from build123d import *

# Parameters (mm, degrees)
F1_DEPTH = 2
F2_DEPTH = 3
F3_R     = 8.2
F4_DEPTH = 7.5
F5_R     = 8.2
F5_R_2   = 7
F6_DEPTH = 20
F7_R     = 9
F7_R_2   = 7
F8_DEPTH = 6.5


with BuildPart() as f1:
    # F0 (on Top) → F1 (new body)
    with BuildSketch(Plane.XY):
        with BuildLine():
            Line((0, 9), (0, 10))
            ThreePointArc((0, 10), (-10, 0), (0, -10))
            Line((0, -10), (0, -9))
            ThreePointArc((0, -9), (-9, 0), (0, 9))
        make_face()
    extrude(amount=F1_DEPTH)

    # F0 (on Top) → F2 (join)
    with BuildSketch(Plane.XY):
        with BuildLine():
            ThreePointArc((0, -10), (7.0710678119, -7.0710678119), (10, 0))
            ThreePointArc((10, 0), (7.0710678119, 7.0710678119), (0, 10))
            Line((0, 10), (0, 9))
            ThreePointArc((0, 9), (6.3639610307, 6.3639610307), (9, 0))
            ThreePointArc((9, 0), (6.3639610307, -6.3639610307), (0, -9))
            Line((0, -9), (0, -10))
        make_face()
    extrude(amount=F2_DEPTH)

    # F3 (on face) → F4 (join)
    with BuildSketch(Plane.XY.offset(2)):
        with BuildLine():
            Line((0, 9), (0, 10))
            ThreePointArc((0, 10), (-10, 0), (0, -10))
            Line((0, -10), (0, -9))
            ThreePointArc((0, -9), (-9, 0), (0, 9))
        make_face()
        with BuildLine():
            ThreePointArc((0, -10), (7.0710678119, -7.0710678119), (10, 0))
            ThreePointArc((10, 0), (7.0710678119, 7.0710678119), (0, 10))
            Line((0, 10), (0, 9))
            ThreePointArc((0, 9), (-9, 0), (0, -9))
            Line((0, -9), (0, -10))
        make_face()
        Circle(F3_R, mode=Mode.SUBTRACT)
    extrude(amount=F4_DEPTH)

    # F5 (on face) → F6 (join)
    with BuildSketch(Plane.XY.offset(9.5)):
        Circle(F5_R)
        Circle(F5_R_2, mode=Mode.SUBTRACT)
    extrude(amount=-F6_DEPTH)

    # F7 (on face) → F8 (cut)
    with BuildSketch(Plane.XY.offset(9.5)):
        Circle(F7_R)
        Circle(F7_R_2, mode=Mode.SUBTRACT)
    extrude(amount=-F8_DEPTH, mode=Mode.SUBTRACT)


solid = f1.part
Design review of the part built by this model. Coordinates are the model's own, in mm. A direction names the side the tool comes from. Coordinates: 2 decimals unless noted, no trailing zeros. Write each loop counter-clockwise with the first axis right and the second up, starting at its lowest first coordinate (ties: lowest second). Pieces come first, ordered by that corner, then holes. Notation, with made-up numbers: (52, -19.5) - (90, -19.5) arc R19 cw to (90, 8.5) - close; hole circle Ø3 at (79.25, -34.5). An arc over 180 degrees is marked (long way). Use one line per item in the form item = value.
Q1. Consider section D-D (z = 7). Write out the cut boundary in (x, y), plus the area to 3 significant figures.
Taken from the geometry:
outline = circle Ø20 at (0, 0); hole circle Ø18 at (0, 0)
area = 59.7 mm^2
Q2. Consider section A-A (z = 1.5). Write out the cut boundary in (x, y).
Taken from the geometry:
outline = circle Ø20 at (0, 0); circle Ø16.4 at (0, 0); hole circle Ø18 at (0, 0); hole circle Ø14 at (0, 0)
Q3. The part is to be moulded in two halves that separate along X. For faces 1 (the flat face through (0, -7.3, 3)), 2 (the cylindrical face through (6.466, -2.681, -3.656)), 3 (the flat face through (-9, 2, 9.5)), 4 (the cylindrical face through (9.54, 3, 4.68)), say which applies: +X half, -X half, draft (parallel to the pull), parting line (faces both ways), or undercut.
Taken from the geometry:
face_1 = undercut
face_2 = undercut
face_3 = draft
face_4 = parting line
Q4. For probe 1 along Y at (x, z) = (0, -2.25); probe 2 along X at (y, z) = (-5.5, 1.5); probe 3 along X at (y, z) = (0.5, 1.75), list the stretches that pass through material, from the lowest coordinate up.
Taken from the geometry:
probe_1 = -8.2 to -7, 7 to 8.2
probe_2 = -8.35 to -7.12, -6.08 to -4.33, 4.33 to 6.08, 7.12 to 8.35
probe_3 = -9.99 to -8.99, -8.18 to -6.98, 6.98 to 8.18, 8.99 to 9.99
Q5. Consider section C-C (y = -1.25). Write out the cut boundary in (x, z), plus the area to 3 significant figures.
Taken from the geometry:
outline = (-9.92, 0) - (-8.91, 0) - (-8.91, 2) - (-8.1, 2) - (-8.1, -10.5) - (-6.89, -10.5) - (-6.89, 3) - (-8.91, 3) - (-8.91, 9.5) - (-9.92, 9.5) - close; (6.89, -10.5) - (8.1, -10.5) - (8.1, 2) - (8.91, 2) - (8.91, 0) - (9.92, 0) - (9.92, 9.5) - (8.91, 9.5) - (8.91, 3) - (6.89, 3) - close
area = 53.6 mm^2
Q6. Machinability: for faces 5 (the flat face through (8, -3, 2)), 6 (the cylindrical face through (-1.172, 8.923, 6.296)), 7 (the flat face through (6, 4, -10.5)), which of the approach directions +Z, -Z, +X, -X, +Y, -Y give a long, thin tool a straight path to every point of the face, cutting with its end or side? Answer none if there is none.
Taken from the geometry:
face_5 = -Z
face_6 = +Z
face_7 = -Z, +X, -X, +Y, -Y
Q7. Consider section B-B (x = 3). Write out the cut boundary in (y, z), plus the area to 3 significant figures.
Taken from the geometry:
outline = (-9.54, 0) - (-8.49, 0) - (-8.49, 2) - (-7.63, 2) - (-7.63, -10.5) - (-6.32, -10.5) - (-6.32, 3) - (-8.49, 3) - (-8.49, 9.5) - (-9.54, 9.5) - close; (6.32, -10.5) - (7.63, -10.5) - (7.63, 2) - (8.49, 2) - (8.49, 0) - (9.54, 0) - (9.54, 9.5) - (8.49, 9.5) - (8.49, 3) - (6.32, 3) - close
area = 57.0 mm^2
Q8. Insertion check: pin 1 Ø1.5 at (x, z) = (-2.5, 7) entering from +Y; pin 2 Ø10 at (x, z) = (0.5, -7) entering from -Y; pin 3 Ø10 at (y, z) = (-5, -8.5) entering from -X; pin 4 Ø6 at (x, y) = (2.5, -2) entering from -Z. Each pin has a flat end and moves straight along its axis. Give the tip position at first contact, or say it passes through.
Taken from the geometry:
pin_1 = 9.85
pin_2 = -8.2
pin_3 = -8.2
pin_4 = through
